from build123d import *

# Parameters (mm, degrees)
F0_W     = 460
F0_H     = 650
F1_DEPTH = 80
F2_W     = 420
F2_H     = 60
F3_DEPTH = 650.001
F4_W     = 600
F4_H     = 2.5
F5_DEPTH = 460.001


with BuildPart() as f1:
    # F0 (on Top) → F1 (new body)
    with BuildSketch(Plane.XY):
        Rectangle(F0_W, F0_H)
    extrude(amount=F1_DEPTH)

    # F2 (on face) → F3 (cut, through all)
    with BuildSketch(Plane.XZ.offset(325)):
        with Locations((0, 30)):
            Rectangle(F2_W, F2_H)
    extrude(amount=-F3_DEPTH, mode=Mode.SUBTRACT)

    # F4 (on face) → F5 (cut, through all)
    with BuildSketch(Plane.YZ.offset(230)):
        with Locations((-25, 21.25)):
            Rectangle(F4_W, F4_H)
    extrude(amount=-F5_DEPTH, mode=Mode.SUBTRACT)


solid = f1.part
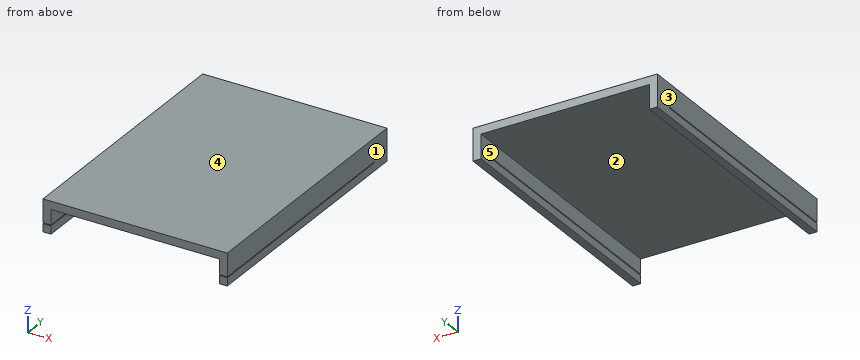
Here's how the part is built. I have some questions about the finished solid (model axes, mm). Face numbers are marked on the shaded views. A direction names the side the tool comes from. Round coordinates to 2 decimals unless told otherwise and drop trailing zeros. Write each loop counter-clockwise with the first axis right and the second up, starting at its lowest first coordinate (ties: lowest second). Pieces come first, ordered by that corner, then holes.
1. Suppose I cut it at A-A (z = 43). List the corners of the cut face in (x, y) for me.
2. Suppose I cut it at C-C (x = -19.5). List the corners of the cut face in (y, z) for me.
3. For the marked faces 4 and 5, which set-ups out of +Z, -Z, +X, -X, +Y, -Y let a thin tool reach every point of the face, with its end or its side?
4. Suppose I cut it at B-B (y = -131). List the corners of the cut face in (x, z) for me.
5. If we mould it in two halves opening along X, with no side actions, what happens to the marked faces 1, 2 and 3? For each: released by +X, released by -X, zero draft, split by the parting line, or undercut.
6. I need wall thicknesses on L1, parallel to X at y = 250, z = 37; L2, parallel to Z at x = -175, y = -287.5. Which ranges of each line are inside material? Lowest first, please.
7. Will this pin go through, and if not, where does the flat tip stop? pin 1 Ø3 at (x, y) = (55, 205.5) entering from -Z.
Answer sheet:
1. outline: (-230, -325) - (-210, -325) - (-210, 325) - (-230, 325) - close; (210, -325) - (230, -325) - (230, 325) - (210, 325) - close
2. outline: (-325, 60) - (325, 60) - (325, 80) - (-325, 80) - close
3. face 4: +Z, +X, -X, +Y, -Y
3. face 5: -Z, +Y, -Y
4. outline: (-230, 0) - (-210, 0) - (-210, 20) - (-230, 20) - close; (-230, 22.5) - (-210, 22.5) - (-210, 60) - (210, 60) - (210, 22.5) - (230, 22.5) - (230, 80) - (-230, 80) - close; (210, 0) - (230, 0) - (230, 20) - (210, 20) - close
5. face 1: released by +X
5. face 2: undercut
5. face 3: released by -X
6. L1: x = -230 to -210, 210 to 230
6. L2: z = 60 to 80
7. pin 1: stops at z = 60
